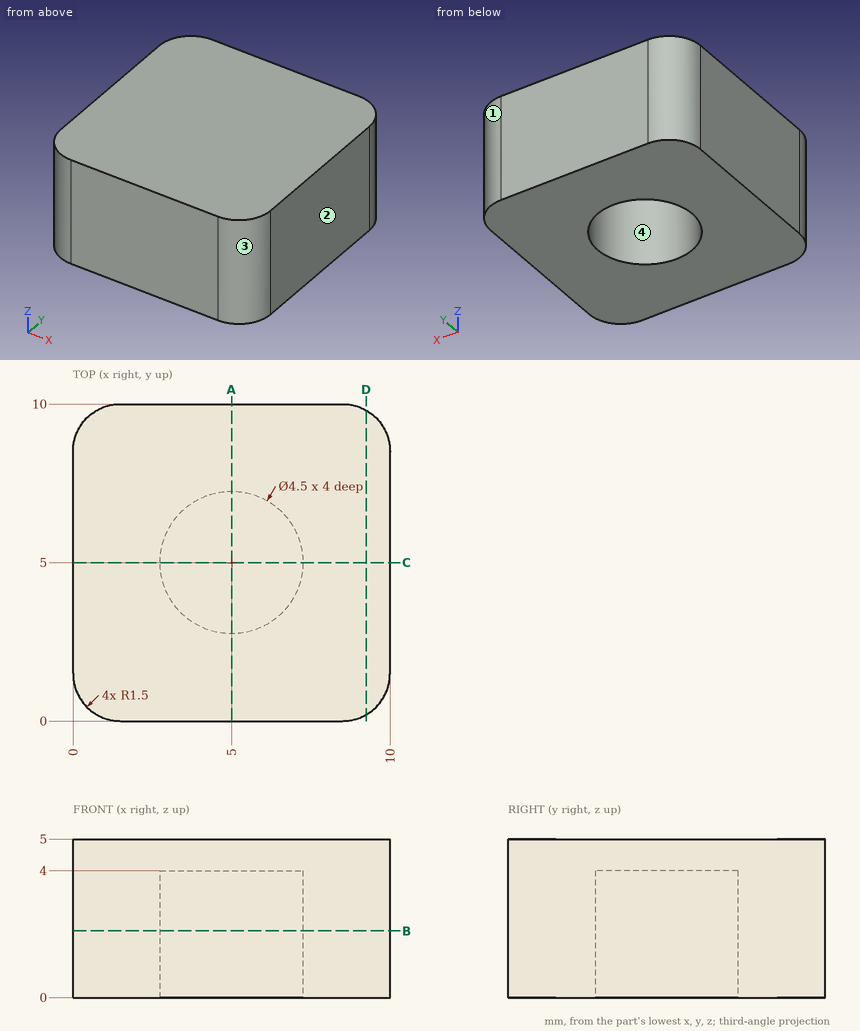
Verification items for this drawing (mm, ordinates from the low corner). Round coordinates to 2 decimals unless told otherwise and drop trailing zeros. Order: outer loops, then holes, each group sorted by start corner. A loop starts at its lowest first (then second) coordinate and runs counter-clockwise, first axis right, second up. Notation, with made-up numbers: M 1.5,-29 L 22.5,-29 A28 cw 22.5,-7 Z; hole C 3,8.5 d1. An arc over 180 degrees is marked long. Answer in a Markdown table with one row per item. Add a question column.
Item 1: Sectioned sample at B-B, the plane z = 2.1. Enter the section's corners in (x, y), plus the area to 3 significant figures.
Item 2: Draft check along Y on the marked faces 1, 2, 3 and 4. Enter one of: released by +Y, released by -Y, zero draft, split by the parting line, or undercut.
Item 3: Sectioned sample at D-D, the plane x = 9.25. Enter the section's corners in (y, z), plus the area to 3 significant figures.
Item 4: Depth check by flat-ended pin: pin 1 Ø2 at (x, y) = (7, 4) entering from -Z; pin 2 Ø2 at (x, y) = (4.5, 5.5) entering from -Z. Enter the tip coordinate at first touch or a pass-through.
Item 5: Sectioned sample at A-A, the plane x = 5. Enter the section's corners in (y, z), plus the area to 3 significant figures.
Item 6: Material ranges on L1, parallel to Y at x = 5, z = 0.9; L2, parallel to Y at x = 3.5, z = 2.1, recorded low to high. Write a range as [from, to].
Filled in:
| question | item | result |
|---|---|---|
| 1 | outline | M 0,1.5 A1.5 ccw 1.5,0 L 8.5,0 A1.5 ccw 10,1.5 L 10,8.5 A1.5 ccw 8.5,10 L 1.5,10 A1.5 ccw 0,8.5 Z; hole C 5,5 d4.5 |
| 1 | area | 82.2 mm² |
| 2 | face 1 | released by +Y |
| 2 | face 2 | zero draft |
| 2 | face 3 | released by -Y |
| 2 | face 4 | undercut |
| 3 | outline | M 0.2,0 L 9.8,0 L 9.8,5 L 0.2,5 Z |
| 3 | area | 48.0 mm² |
| 4 | pin 1 | stops at z = 0 |
| 4 | pin 2 | stops at z = 4 |
| 5 | outline | M 0,0 L 2.75,0 L 2.75,4 L 7.25,4 L 7.25,0 L 10,0 L 10,5 L 0,5 Z |
| 5 | area | 32.0 mm² |
| 6 | L1 | y = [0, 2.75], [7.25, 10] |
| 6 | L2 | y = [0, 3.32], [6.68, 10] |
